Verification items for this drawing (mm, ordinates from the low corner). A direction names the side the tool comes from. Coordinates: 2 decimals unless noted, no trailing zeros. Loops run counter-clockwise (first coordinate to the right, second up) from the corner with the lowest first, then second, coordinate; pieces in that order, holes last. Notation, with made-up numbers: (86, -5.75) - (107, -5.75) arc R23 ccw to (107, 26.25) - close; hole circle Ø11 at (46.5, 76). An arc over 180 degrees is marked (long way). Write each question's results on one line, items separated by ' | '. Start each with the question number.
(1) Access from +Z, -Z, +X, -X, +Y, -Y to the whole of each face (thin tool, end or side, straight path). Record for the marked faces 1, 2, 3, 4 and 5.
(2) Material ranges on probe 1 along X at (y, z) = (4, 42); probe 2 along Z at (x, y) = (97, 16.25); probe 3 along X at (y, z) = (16, 24), recorded low to high.
(3) Sectioned sample at B-B (x = 94). Enter the section's corners in (y, z).
(4) Sectioned sample at D-D (y = 12). Enter the section's corners in (x, z).
(5) Sectioned sample at A-A (y = 19.5). Enter the section's corners in (x, z).
(6) Sectioned sample at C-C (z = 52.5). Enter the section's corners in (x, y), plus the area to 3 significant figures.
(7) Go/stop test with flat-tipped pins: pin 1 Ø12 at (x, y) = (69.5, 14.5) entering from -Z; pin 2 Ø1.5 at (x, z) = (14, 23) entering from -Y; pin 3 Ø9 at (x, y) = (15, 14) entering from +Z; pin 4 Ø9.5 at (x, z) = (16, 30.5) entering from -Y. Record where each tip stops, or that it passes through.
(8) Mould release check, pull along Z, two halves, no side actions. Record for the marked faces 6, 7 and 8: pulls with the +Z half, pulls with the -Z half, needs draft (parallel to the pull), parting line crosses it, or undercut.
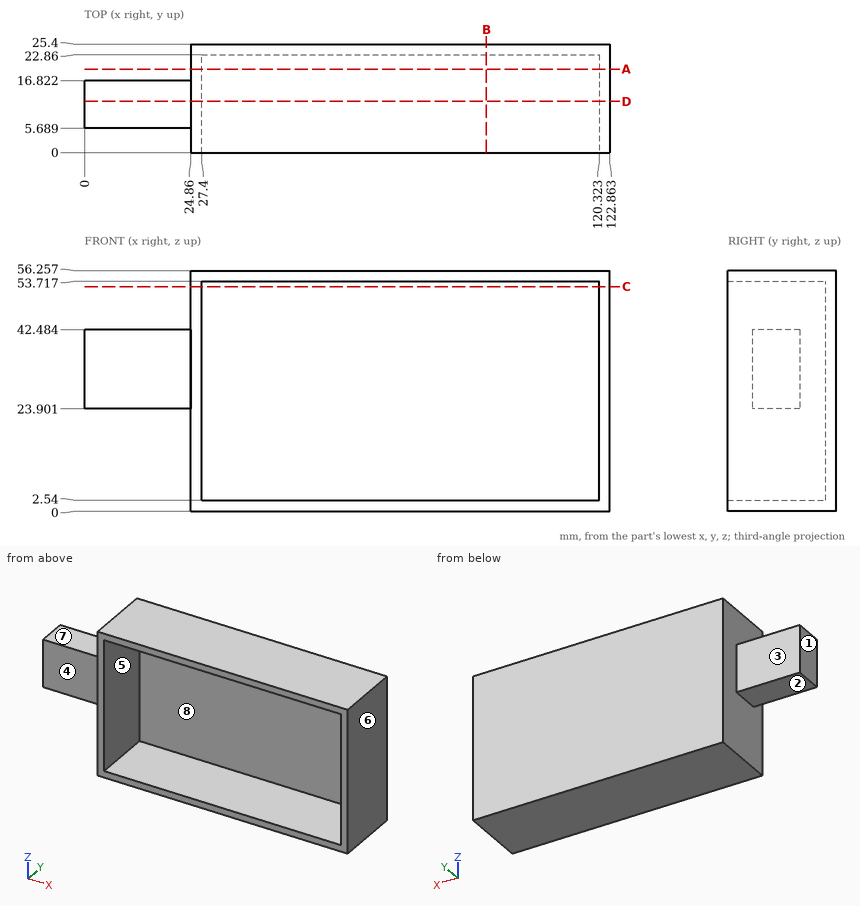
Outcome:
1) face 1: +Z, -Z, -X, +Y, -Y | face 2: -Z, -X, +Y, -Y | face 3: +Z, -Z, -X, +Y | face 4: +Z, -Z, -X, -Y | face 5: -Y
2) probe 1: x = 24.86 to 27.4, 120.32 to 122.86 | probe 2: z = 0 to 2.54, 53.72 to 56.26 | probe 3: x = 0 to 27.4, 120.32 to 122.86
3) outline: (0, 0) - (25.4, 0) - (25.4, 56.26) - (0, 56.26) - (0, 53.72) - (22.86, 53.72) - (22.86, 2.54) - (0, 2.54) - close
4) outline: (0, 23.9) - (24.86, 23.9) - (24.86, 0) - (122.86, 0) - (122.86, 56.26) - (24.86, 56.26) - (24.86, 42.48) - (0, 42.48) - close; hole (27.4, 2.54) - (120.32, 2.54) - (120.32, 53.72) - (27.4, 53.72) - close
5) outline: (24.86, 0) - (122.86, 0) - (122.86, 56.26) - (24.86, 56.26) - close; hole (27.4, 2.54) - (120.32, 2.54) - (120.32, 53.72) - (27.4, 53.72) - close
6) outline: (24.86, 0) - (27.4, 0) - (27.4, 22.86) - (120.32, 22.86) - (120.32, 0) - (122.86, 0) - (122.86, 25.4) - (24.86, 25.4) - close | area: 365 mm2
7) pin 1: stops at z = 0 | pin 2: passes through | pin 3: stops at z = 42.48 | pin 4: stops at y = 5.69
8) face 6: needs draft | face 7: pulls with the +Z half | face 8: undercut
